```python
from build123d import *

# Parameters (mm, degrees)
F0_W     = 31.75
F0_H     = 165.1
F1_DEPTH = 5.08
F2_DEPTH = 19.05
F3_R     = 5.08
F4_DEPTH = 45.72


with BuildPart() as f1:
    # F0 (on Top) → F1 (new body)
    with BuildSketch(Plane.XY):
        with Locations((-29.231615, -10.24527)):
            Rectangle(F0_W, F0_H)
    extrude(amount=F1_DEPTH)

    # F0 (on Top) → F2 (join)
    with BuildSketch(Plane.XY):
        Polygon((-45.106615, -92.79527), (-45.106615, 72.30473), (-51.456615, 78.65473), (-51.456615, -99.14527), (-7.006615, -99.14527), (-7.006615, 78.65473), (-13.356615, 72.30473), (-13.356615, -92.79527), align=None)
    extrude(amount=F2_DEPTH)

    # F3 (on face) → F4 (cut)
    with BuildSketch(Plane.YZ.offset(-7.006615)):
        with Locations((-84.609412, 12.154419)):
            Circle(F3_R)
    extrude(amount=-F4_DEPTH, mode=Mode.SUBTRACT)


solid = f1.part
```
The listing builds one solid part. Answer for the finished solid, in the listing's coordinates (mm). A direction names the side the tool comes from. Give positions to 0.01 mm unless a question says otherwise; leave off trailing zeros. Loops run counter-clockwise (first coordinate to the right, second up) from the corner with the lowest first, then second, coordinate; pieces in that order, holes last. Notation, with made-up numbers: (70, -10.5) - (77, -10.5) arc R30 cw to (77, 21.5) - close; hole circle Ø9 at (-11.75, 43.5). An arc over 180 degrees is marked (long way). Answer as CSV lines item,"result". Start each with the question number.
Item 1: A cutting plane is placed at D-D on x = -21.5. Determine the outline of the cut face in (y, z), then the cut area to 3 significant figures.
Item 2: A cutting plane is placed at B-B on z = 8.75. Determine the outline of the cut face in (x, y), then the cut area to 3 significant figures.
Item 3: For faces 4 (the face through (-13.357, -9, 12)), 5 (the face through (-10.137, -89.684, 12.378)), 6 (the face through (-29, 72.305, 3)), determine the directions among +Z, -Z, +X, -X, +Y, -Y from which every point of the face is accessible in a straight line to the end or side of a thin tool.
Item 4: Find the intervals of material crossed by line 1 (X direction, y = 50, z = 14); line 2 (Y direction, x = -26, z = 2.5); line 3 (Z direction, x = -15, y = -12), in increasing order. Write a range as from..to.
Item 5: A cutting plane is placed at C-C on y = -84.5. Determine the outline of the cut face in (x, z), then the cut area to 3 significant figures.
Item 6: The mould has two halves that part along Z. Classify faces 1 (the face through (-29, -9, 5.08)), 2 (the face through (-51.457, -9, 9)), 3 (the face through (-48.237, -89.684, 12.378)): +Z half, -Z half, draft (parallel to the pull), parting line (faces both ways), or undercut.
Item 7: A cutting plane is placed at A-A on y = -20.5. Determine the outline of the cut face in (x, z), then the cut area to 3 significant figures.
Item 8: Each of these flat-tipped pins is pushed along its axis until it touches: pin 1 (5 mm diameter, centred on x = -39, y = -6, fed in from +Z); pin 2 (4 mm diameter, centred on x = -37.5, z = 15, fed in from +Y); pin 3 (8 mm diameter, centred on y = -84.61, z = 12.15, fed in from -X); pin 4 (12 mm diameter, centred on x = -12.5, y = 14, fed in from -Z). Where does it stop, or does it pass through?
Found:
1,outline,"(-99.15, 0) - (72.3, 0) - (72.3, 5.08) - (-92.8, 5.08) - (-92.8, 19.05) - (-99.15, 19.05) - close"
1,area,"960 mm^2"
2,outline,"(-51.46, -99.15) - (-7.01, -99.15) - (-7.01, -88.38) - (-13.36, -88.38) - (-13.36, -92.8) - (-45.11, -92.8) - (-45.11, -88.38) - (-51.46, -88.38) - close; (-51.46, -80.84) - (-45.11, -80.84) - (-45.11, 72.3) - (-51.46, 78.65) - close; (-13.36, -80.84) - (-7.01, -80.84) - (-7.01, 78.65) - (-13.36, 72.3) - close"
2,area,"2,320 mm^2"
3,face 4,"+Z, +Y"
3,face 5,"+X, -X"
3,face 6,"+Z, -Z, +Y"
4,line 1,"x = -51.46..-45.11, -13.36..-7.01"
4,line 2,"y = -99.15..72.3"
4,line 3,"z = 0..5.08"
5,outline,"(-51.46, 0) - (-7.01, 0) - (-7.01, 7.08) - (-13.36, 7.08) - (-13.36, 5.08) - (-45.11, 5.08) - (-45.11, 7.08) - (-51.46, 7.08) - close; (-51.46, 17.23) - (-45.11, 17.23) - (-45.11, 19.05) - (-51.46, 19.05) - close; (-13.36, 17.23) - (-7.01, 17.23) - (-7.01, 19.05) - (-13.36, 19.05) - close"
5,area,"274 mm^2"
6,face 1,"+Z half"
6,face 2,"draft"
6,face 3,"undercut"
7,outline,"(-51.46, 0) - (-7.01, 0) - (-7.01, 19.05) - (-13.36, 19.05) - (-13.36, 5.08) - (-45.11, 5.08) - (-45.11, 19.05) - (-51.46, 19.05) - close"
7,area,"403 mm^2"
8,pin 1,"stops at z = 5.08"
8,pin 2,"stops at y = -92.8"
8,pin 3,"passes through"
8,pin 4,"stops at z = 0"
